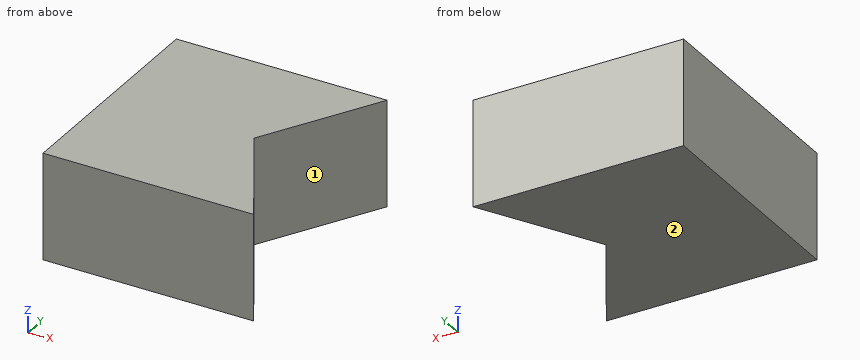
from build123d import *

# Parameters (mm, degrees)
CROQUIS1_R                 = 1.5
SALIENTE_EXTRUIR1_DEPTH    = 7
CORTAR_EXTRUIR1_DEPTH      = 10
CORTAR_EXTRUIR1_DEPTH_BACK = 27.438608133
CROQUIS2_R                 = 1.5
CORTAR_EXTRUIR2_DEPTH      = 27.438608133
CORTAR_EXTRUIR2_DEPTH_BACK = 27.438608133
CROQUIS3_W                 = 6
CROQUIS3_H                 = 7
CORTAR_EXTRUIR3_DEPTH      = 1.5
CROQUIS5_OUTSIDE_W         = 50.708
CROQUIS5_OUTSIDE_H         = 20.708
CROQUIS5_OUTSIDE_W_2       = 3
CROQUIS5_OUTSIDE_H_2       = 6
CORTAR_EXTRUIR4_DEPTH      = 27.438608133
CROQUIS6_OUTSIDE_W         = 6.706
CROQUIS6_OUTSIDE_H         = 9.706
CROQUIS6_OUTSIDE_W_2       = 2.6
CROQUIS6_OUTSIDE_H_2       = 5.6
CORTAR_EXTRUIR5_DEPTH      = 7.245101176


with BuildPart() as part:
    # Croquis1 → Saliente-Extruir1 (new, symmetric)
    with BuildSketch(Plane(origin=(0, 0, 0), x_dir=(0, 0, -1), z_dir=(1, 0, 0))):
        with BuildLine():
            Line((-24, 5), (15, 5))
            Line((15, 5), (15, -5))
            Line((15, -5), (-24, -5))
            ThreePointArc((-24, -5), (-24.707106781, -4.707106781), (-25, -4))
            Line((-25, -4), (-25, 4))
            ThreePointArc((-25, 4), (-24.707106781, 4.707106781), (-24, 5))
        make_face()
        with Locations((-22, 0)):
            Circle(CROQUIS1_R, mode=Mode.SUBTRACT)
    extrude(amount=SALIENTE_EXTRUIR1_DEPTH, both=True)

    # Croquis2 → Cortar-Extruir1 (cut, two sides: drawn at the far end of the back side and taken through both)
    with BuildSketch(Plane.XY.offset(-CORTAR_EXTRUIR1_DEPTH_BACK)):
        Circle(CROQUIS2_R)
    extrude(amount=CORTAR_EXTRUIR1_DEPTH + CORTAR_EXTRUIR1_DEPTH_BACK, mode=Mode.SUBTRACT)

    # Croquis3 → Cortar-Extruir2 (cut, two sides: drawn at the far end of the back side and taken through both)
    with BuildSketch(Plane(origin=(0, 0, 0), x_dir=(1, 0, 0), z_dir=(0, 1, 0)).offset(-CORTAR_EXTRUIR2_DEPTH_BACK)):
        with Locations((0, -21.5)):
            Rectangle(CROQUIS3_W, CROQUIS3_H)
    extrude(amount=CORTAR_EXTRUIR2_DEPTH + CORTAR_EXTRUIR2_DEPTH_BACK, mode=Mode.SUBTRACT)

    # Croquis4 → Cortar-Extruir3 (cut, symmetric)
    with BuildSketch(Plane.XY):
        Polygon((1.732050808, 3), (-1.732050808, 3), (-3.464101615, 0), (-1.732050808, -3), (1.732050808, -3), (3.464101615, 0), align=None)
    extrude(amount=CORTAR_EXTRUIR3_DEPTH, both=True, mode=Mode.SUBTRACT)

    # Croquis5 outside → Cortar-Extruir4 (cut, through all)
    with BuildSketch(Plane(origin=(0, 0, 0), x_dir=(0, 0, -1), z_dir=(1, 0, 0))):
        with Locations((-5, 0)):
            Rectangle(CROQUIS5_OUTSIDE_W, CROQUIS5_OUTSIDE_H)
        Rectangle(CROQUIS5_OUTSIDE_W_2, CROQUIS5_OUTSIDE_H_2, mode=Mode.SUBTRACT)
    extrude(amount=-CORTAR_EXTRUIR4_DEPTH, mode=Mode.SUBTRACT)


with BuildPart() as body_2:
    # of the pieces the cut leaves, the one that is kept (cortar_extruir4_keep)
    add(part.part.solids().sort_by_distance((-7, 3, -1.5))[0])

    # Croquis6 outside → Cortar-Extruir5 (cut, through all)
    with BuildSketch(Plane.ZY.offset(7)):
        Rectangle(CROQUIS6_OUTSIDE_W, CROQUIS6_OUTSIDE_H)
        Rectangle(CROQUIS6_OUTSIDE_W_2, CROQUIS6_OUTSIDE_H_2, mode=Mode.SUBTRACT)
    extrude(amount=-CORTAR_EXTRUIR5_DEPTH, mode=Mode.SUBTRACT)


solid = body_2.part
Geometry check sheet. Reference: the model listing, model coordinates, mm. Face numbers are marked on the shaded views. A direction names the side the tool comes from. Give positions to 0.01 mm unless a question says otherwise; leave off trailing zeros. Write each loop counter-clockwise with the first axis right and the second up, starting at its lowest first coordinate (ties: lowest second). Pieces come first, ordered by that corner, then holes.
1) Cross-section at C-C (x = -2.95). Record the boundary of the cut face in (y, z), plus the area to 3 significant figures.
Values follow:
outline: (-2.8, -1.3) - (-0.89, -1.3) - (-0.89, 1.3) - (-2.8, 1.3) - close; (0.89, -1.3) - (2.8, -1.3) - (2.8, 1.3) - (0.89, 1.3) - close
area: 9.93 mm2
2) Cross-section at A-A (x = -2.4). Record the boundary of the cut face in (y, z), plus the area to 3 significant figures.
Values follow:
outline: (-2.8, -1.3) - (-1.84, -1.3) - (-1.84, 1.3) - (-2.8, 1.3) - close; (1.84, -1.3) - (2.8, -1.3) - (2.8, 1.3) - (1.84, 1.3) - close
area: 4.98 mm2
3) Set-up check for the marked faces 1 and 2: record each of +Z, -Z, +X, -X, +Y, -Y from which the full face is reachable in a straight line by a thin tool's end or side.
Values follow:
face 1: +Z, -Z, +X
face 2: -Z, +X, -X, +Y, -Y
4) Thickness scan on line 1 (Y direction, x = -2.05, z = -1); line 2 (X direction, y = 1.15, z = -0.8); line 3 (Y direction, x = -2.4, z = 1). Record the ranges inside material, lowest first.
Values follow:
line 1: y = -2.8 to -2.45, 2.45 to 2.8
line 2: x = -7 to -2.8
line 3: y = -2.8 to -1.84, 1.84 to 2.8
5) Cross-section at B-B (z = 0.5). Record the boundary of the cut face in (x, y).
Values follow:
outline: (-7, -2.8) - (-1.85, -2.8) - (-3.46, 0) - (-1.85, 2.8) - (-7, 2.8) - close
6) Cross-section at D-D (y = 1.2). Record the boundary of the cut face in (x, z), plus the area to 3 significant figures.
Values follow:
outline: (-7, -1.3) - (-2.77, -1.3) - (-2.77, 1.3) - (-7, 1.3) - close
area: 11.0 mm2
